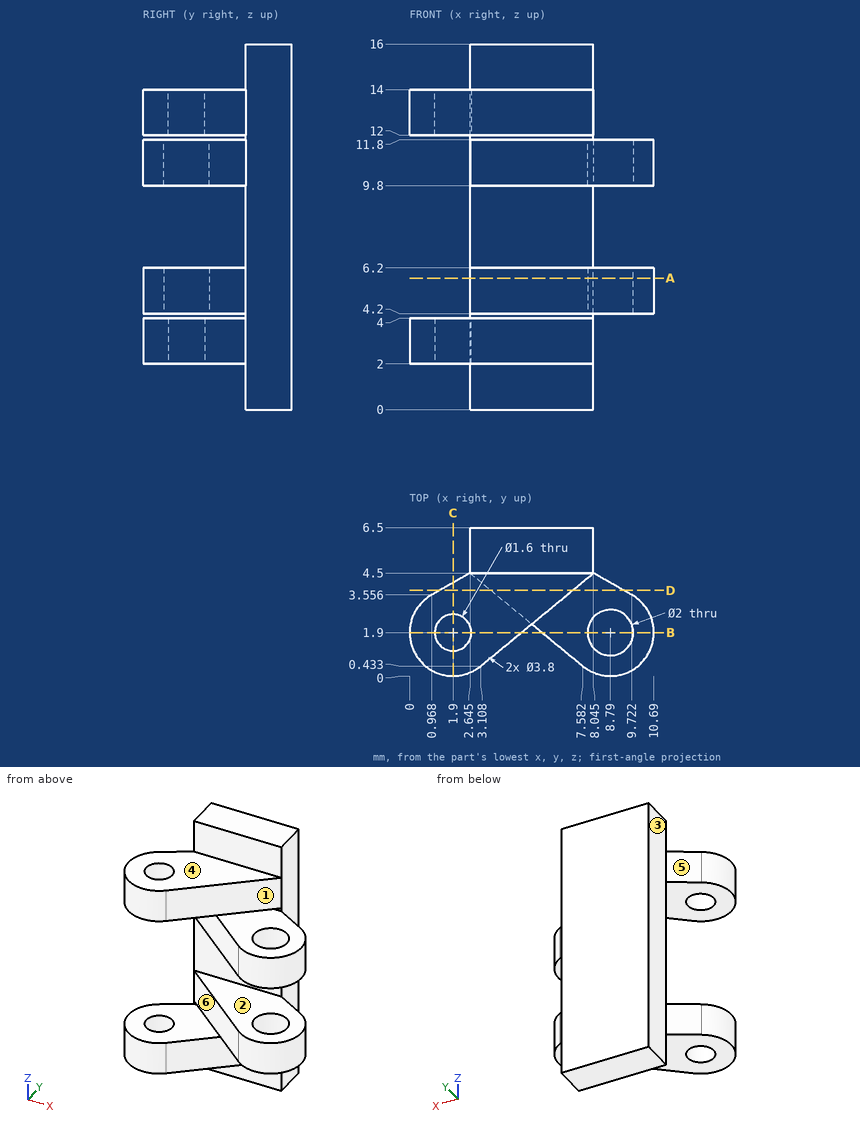
Geometry: see drawing. Coordinates: mm, zero at the bounding-box minimum. A direction names the side the tool comes from. Coordinates: 2 decimals unless noted, no trailing zeros. Write each loop counter-clockwise with the first axis right and the second up, starting at its lowest first coordinate (ties: lowest second). Pieces come first, ordered by that corner, then holes. Notation, with made-up numbers: M 75,57.25 L 91,57.25 A26 cw 91,91.25 Z; hole C 27,62 d11. An arc over 180 degrees is marked long. Answer as a JSON object with one key per item and string values.
1. Ray query, L1, parallel to Z at x = 6.75, y = 4; L2, parallel to Z at x = 2.75, y = 1.5; L3, parallel to Z at x = 6.75, y = 2.5. Return the intervals inside material, ascending.
Evaluation:
{"L1": "2 to 4, 4.2 to 6.2, 9.8 to 11.8, 12 to 14", "L2": "2 to 4, 12 to 14", "L3": "4.2 to 6.2, 9.8 to 11.8"}
2. Cut plane B-B on y = 1.9. State how many separate pieces and enclosed holes the cut face has.
Evaluation:
{"separate pieces": "8", "enclosed holes": "0"}
3. Contact query for flat-ended pins moving along their axis: P1, Ø1.5, axis at y = 1, z = 2, coming from the +X side (1 decimal); P2, Ø1.6, axis at x = 6, z = 15, coming from the -Y side; P3, Ø2, axis at y = 6, z = 8.5, coming from the +X side (3 decimals). Output: stop coordinate, or through.
Evaluation:
{"P1": "x = 4.7", "P2": "y = 4.5", "P3": "x = 8.045"}
4. Cut plane A-A on z = 5.75. Output: boundary loops of the cut face in (x, y) (1 decimal).
Evaluation:
{"outline": "M 2.6,4.5 L 7.6,0.4 A1.9 ccw long 9.7,3.6 L 8,4.5 L 8,6.5 L 2.6,6.5 Z; hole C 8.8,1.9 d2"}
5. Draft query along Z for the marked faces 4, 5 and 6. Return one class per face: released by +Z, released by -Z, zero draft, split by the parting line, or undercut.
Evaluation:
{"face 4": "released by +Z", "face 5": "zero draft", "face 6": "undercut"}
6. Access query for the marked faces 1, 2 and 3. Directions: +Z, -Z, +X, -X, +Y, -Y. A direction counts if a zero-diameter tool reaches every point of the face in a straight line with its end or side. Return the directions, or none.
Evaluation:
{"face 1": "+Z, +X, -Y", "face 2": "+X, -X, -Y", "face 3": "+Z, -Z, -X, +Y"}
7. Cut plane C-C on x = 1.9. Output: boundary loops of the cut face in (y, z).
Evaluation:
{"outline": "M 0,2 L 1.1,2 L 1.1,4 L 0,4 Z; M 0,12 L 1.1,12 L 1.1,14 L 0,14 Z; M 2.7,2 L 4.08,2 L 4.08,4 L 2.7,4 Z; M 2.7,12 L 4.08,12 L 4.08,14 L 2.7,14 Z"}
8. Cut plane D-D on y = 3.75. Output: boundary loops of the cut face in (x, z) (1 decimal).
Evaluation:
{"outline": "M 1.3,2 L 7.1,2 L 7.1,4 L 1.3,4 Z; M 1.3,12 L 7.1,12 L 7.1,14 L 1.3,14 Z; M 3.6,4.2 L 9.4,4.2 L 9.4,6.2 L 3.6,6.2 Z; M 3.6,9.8 L 9.4,9.8 L 9.4,11.8 L 3.6,11.8 Z"}
